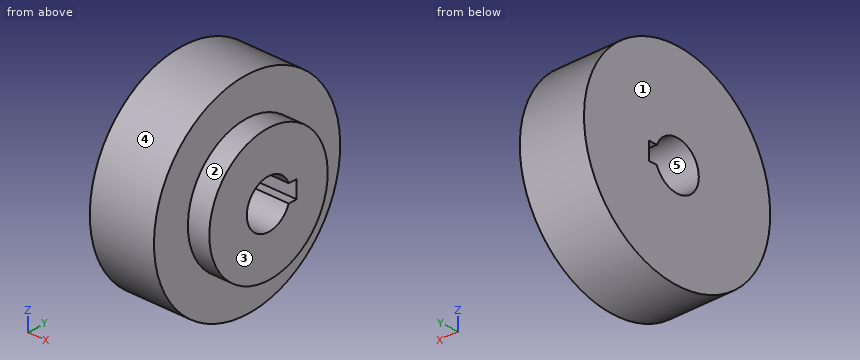
```python
from build123d import *

# Parameters (mm, degrees)
SKETCH2_W          = 8
SKETCH2_H          = 6.6
CUT_EXTRUDE1_DEPTH = 78.787924834


with BuildPart() as part:
    # Sketch1 → Revolve1 (revolve)
    with BuildSketch(Plane.XY, mode=Mode.PRIVATE) as revolve1_sk:
        Polygon((0, 11), (0, 47.175), (30, 47.175), (30, 30), (40, 30), (40, 11), align=None)
    revolve(revolve1_sk.sketch.rotate(Axis((0, 0, 0), (1, 0, 0)), 90), axis=Axis((0, 0, 0), (1, 0, 0)))

    # Sketch2 → Cut-Extrude1 (cut, through all)
    with BuildSketch(Plane.ZY):
        with Locations((0, 11)):
            Rectangle(SKETCH2_W, SKETCH2_H)
    extrude(amount=-CUT_EXTRUDE1_DEPTH, mode=Mode.SUBTRACT)


solid = part.part
```
For this review, take the finished solid that the model builds, in its own axes (mm). Face numbers are marked on the shaded views. A direction names the side the tool comes from. Coordinates: 2 decimals unless noted, no trailing zeros. Loops run counter-clockwise (first coordinate to the right, second up) from the corner with the lowest first, then second, coordinate; pieces in that order, holes last. Notation, with made-up numbers: (-15, -1) -> (-3, -1) arc R21 cw to (-3, 19) -> close; hole circle Ø7 at (-11.5, 52.25). An arc over 180 degrees is marked (long way). Return JSON: item names as keys, results as strings. Group by question number.
(1) Consider section C-C, the plane x = 36. Give the boundary of the cut face in (y, z).
(2) Consider section A-A, the plane y = 0. Give the boundary of the cut face in (x, z) (3 decimals), plus the area to 3 significant figures.
(3) Consider section B-B, the plane z = 0. Give the boundary of the cut face in (x, y) (3 decimals).
(4) For pin 1 Ø10 at (x, z) = (32, -12) entering from +Y; pin 2 Ø12 at (x, y) = (31.5, 34.5) entering from -Z; pin 3 Ø6 at (y, z) = (-9.5, 36) entering from +X, all flat-tipped, find the tip position at first contact; note any pin that passes through.
(5) Consider section D-D, the plane z = -18. Give the boundary of the cut face in (x, y).
(6) To check wall thickness, follow L1, parallel to Y at x = 12.5, z = 0 (3 decimals); L2, parallel to X at y = 9, z = -35.5; L3, parallel to Z at x = 17, y = -8. State the ranges of each line that lie inside material, in increasing order.
(7) Tool access review of the marked faces 1 and 2: name each direction out of +Z, -Z, +X, -X, +Y, -Y from which nothing blocks a thin tool from reaching the whole face with its end or side.
(8) Mouldability with a two-part tool opening along Y and no side actions: class the marked faces 3, 4 and 5 as pulls with the +Y half, pulls with the -Y half, needs draft (parallel to the pull), parting line crosses it, or undercut.
Results below:
{
 "1": {"outline": "circle Ø60 at (0, 0); hole (10.25, -4) -> (14.3, -4) -> (14.3, 4) -> (10.25, 4) arc R11 ccw (long way) to start"},
 "2": {"outline": "(0, -47.175) -> (30, -47.175) -> (30, -30) -> (40, -30) -> (40, -11) -> (0, -11) -> close; (0, 11) -> (40, 11) -> (40, 30) -> (30, 30) -> (30, 47.175) -> (0, 47.175) -> close", "area": "2,550 mm2"},
 "3": {"outline": "(0, -47.175) -> (30, -47.175) -> (30, -30) -> (40, -30) -> (40, -11) -> (0, -11) -> close; (0, 14.3) -> (40, 14.3) -> (40, 30) -> (30, 30) -> (30, 47.175) -> (0, 47.175) -> close"},
 "4": {"pin 1": "stops at y = 46.59", "pin 2": "stops at z = -37.45", "pin 3": "stops at x = 30"},
 "5": {"outline": "(0, -43.61) -> (30, -43.61) -> (30, -24) -> (40, -24) -> (40, 24) -> (30, 24) -> (30, 43.61) -> (0, 43.61) -> close"},
 "6": {"L1": "y = -47.175 to -11, 14.3 to 47.175", "L2": "x = 0 to 30", "L3": "z = -46.49 to -7.55, 7.55 to 46.49"},
 "7": {"face 1": "+Z, -Z, -X, +Y, -Y", "face 2": "+X"},
 "8": {"face 3": "needs draft", "face 4": "parting line crosses it", "face 5": "undercut"}
}
